Autodesk Inventor part; units mm, degrees
ref_plane "Work Plane1" through (-21.8189, 29, 8.1) normal (0, 1, 0) x (0, 0, 1)
ref_plane "Work Plane2" through (-21.8189, 19, 8.1) normal (0, 0, -1) x (0, 1, 0)
ref_plane "YZ Plane" through (0, 0, 0) normal (1, 0, 0) x (0, 1, 0)
sketch "Sketch1" plane through (0, 0, 0) normal (0, 0, 1) x (1, 0, 0)
  line L0 (5.8439, -14.5) -> (6.8, -14.5)
  line L1 (6.8, -5.5) -> (6.8, -14.5)
  line L2 (6.8, -5.5) -> (5.8439, -5.5)
  arc A0 (5.8439, -3.1) -> (5.8439, -5.5) centre (4, -4.3) ccw
  line L3 (5.8439, -3.1) -> (6.8, -3.1)
  line L4 (6.8, 0) -> (6.8, -3.1)
  line L5 (0, 0) -> (6.8, 0)
  line L6 (0, -20) -> (0, 0)
  line L7 (0, -20) -> (6.8, -20)
  line L8 (6.8, -16.9) -> (6.8, -20)
  line L9 (6.8, -16.9) -> (5.8439, -16.9)
  arc A1 (5.8439, -14.5) -> (5.8439, -16.9) centre (4, -15.7) ccw
  line L10 (-47.1, -14.5) -> (-46.1439, -14.5)
  arc A2 (-46.1439, -16.9) -> (-46.1439, -14.5) centre (-44.3, -15.7) ccw
  line L11 (-46.1439, -16.9) -> (-47.1, -16.9)
  line L12 (-47.1, -16.9) -> (-47.1, -20)
  line L13 (-40.3, -20) -> (-47.1, -20)
  line L14 (-40.3, 0) -> (-40.3, -20)
  line L15 (-40.3, 0) -> (-47.1, 0)
  line L16 (-47.1, 0) -> (-47.1, -3.1)
  line L17 (-47.1, -3.1) -> (-46.1439, -3.1)
  arc A3 (-46.1439, -5.5) -> (-46.1439, -3.1) centre (-44.3, -4.3) ccw
  line L18 (-46.1439, -5.5) -> (-47.1, -5.5)
  line L19 (-47.1, -5.5) -> (-47.1, -14.5)
extrude "Extrusion1" add sketch "Sketch1" along normal blind 4
sketch "Sketch2" plane through (0, 0, 0) normal (0, 1, 0) x (1, 0, 0)
  line L0 (0, 0) -> (6.8, 0)
  line L1 (0, 0) -> (0, -4)
  line L2 (6.8, -4) -> (0, -4)
  line L3 (6.8, 0) -> (6.8, -4)
  line L4 (-47.1, 0) -> (-47.1, -4)
  line L5 (-40.3, -4) -> (-47.1, -4)
  line L6 (6.8, 0) -> (-47.1, 0)
  line L7 (-47.1, 0) -> (-47.1, -4)
  line L8 (-47.1, -4) -> (6.8, -4)
  line L9 (6.8, -4) -> (6.8, 0)
extrude "Extrusion2" add sketch "Sketch2" along normal blind 4 contours L1 L8 L5 L4 L6
sketch "Sketch3" plane through (0, 0, 4) normal (1, 0, 0) x (0, 0, -1)
  line L0 (4, 0) -> (0, 0)
  line L1 (4, 4) -> (4, 0)
  line L2 (0, 4) -> (4, 4)
  line L3 (0, 0) -> (0, 4)
extrude "Extrusion3" add sketch "Sketch3" along normal up to surface (6.8 mm away)
sketch "Sketch4" plane through (0, 4, 0) normal (0, 1, 0) x (1, 0, 0)
  line L0 (6.8, 0) -> (-47.1, 0)
  line L1 (-47.1, -4) -> (6.8, -4)
  line L2 (-9.3767, -8.1) -> (-9.3767, -13.1) construction
  line L3 (-21.8189, -8.1) -> (-9.3767, -8.1) construction
  arc A0 (-17.3767, -8.1) -> (-40.8, 16.4941) centre (-48.3, -14.1) ccw construction
  line L4 (-9.3767, -4) -> (-16.3767, -4) construction
  line L5 (-16.3767, -4) -> (-16.3767, -8.1) construction
  line L6 (-16.3767, -8.1) -> (-9.3767, -8.1) construction
  line L7 (-9.3767, -8.1) -> (-9.3767, -4) construction
  line L8 (-9.3767, -4) -> (-16.3767, -4)
  line L9 (-16.3767, -4) -> (-16.3767, 0)
  line L10 (-16.3767, 0) -> (-9.3767, 0)
  line L11 (-9.3767, 0) -> (-9.3767, -4)
  point P0 (0, 0)
  dimension "d6" = 7
ref_plane "Work Plane1" through (-21.8189, 29, 8.1) normal (0, 1, 0) x (0, 0, 1)
extrude "Extrusion4" add sketch "Sketch4" along normal up to surface (25 mm away)
sketch "Sketch5" plane through (0, 0, 4) normal (0, 0, 1) x (1, 0, 0)
  circle A0 centre (-13.3767, 24) radius 2 construction
  line L0 (-21.8189, 24) -> (-17.3767, 24) construction
  line L1 (-21.8189, 24) -> (-21.8189, 29) construction
  line L2 (-21.8189, 29) -> (-9.3767, 29) construction
  line L3 (-9.3767, 19) -> (-9.3767, 29) construction
  line L4 (-17.3767, 19) -> (-9.3767, 19) construction
  line L5 (-17.3767, 24) -> (-17.3767, 19) construction
  line L6 (-9.3767, 19) -> (-16.3767, 19) construction
  line L7 (-16.3767, 19) -> (-16.3767, 29) construction
  line L8 (-16.3767, 29) -> (-9.3767, 29) construction
  line L9 (-9.3767, 29) -> (-9.3767, 19) construction
  line L10 (-9.3767, 19) -> (-16.3767, 19)
  line L11 (-16.3767, 19) -> (-16.3767, 29)
  line L12 (-16.3767, 29) -> (-9.3767, 29)
  line L13 (-9.3767, 29) -> (-9.3767, 19)
  circle A1 centre (-13.3767, 24) radius 2
ref_plane "Work Plane2" through (-21.8189, 19, 8.1) normal (0, 0, -1) x (0, 1, 0)
extrude "Extrusion5" add sketch "Sketch5" along normal up to surface (4.1 mm away)
sketch "Sketch6" plane through (-16.3767, 19, 8.1) normal (-1, 0, 0) x (0, 0, 1)
  line L0 (0, 5) -> (-24.5941, 5) construction
  line L1 (0, 0) -> (-24.5941, 0) construction
  line L2 (-8.1, 10) -> (0.5132, 10) construction
  line L3 (0.5132, 10) -> (0.5132, 5) construction
  line L4 (0.5132, 5) -> (-8.1, 5) construction
  line L5 (-8.1, 5) -> (-8.1, 10) construction
  line L6 (-8.1, 10) -> (0, 10)
  line L7 (0, 10) -> (0, 5)
  line L8 (0, 5) -> (-8.1, 5)
  line L9 (-8.1, 5) -> (-8.1, 10)
  point P0 (-8.1, -19)
extrude "Extrusion6" add sketch "Sketch6" along normal blind 5
sketch "Sketch7" plane through (-16.3767, 24, 0) normal (0, -1, 0) x (1, 0, 0)
  line L0 (0, 8.1) -> (0, 0)
  line L1 (0, 8.1) -> (-5, 8.1)
  line L2 (-5, 0) -> (-5, 8.1)
  line L3 (0, 0) -> (-5, 0)
  point P0 (16.3767, 0)
extrude "Extrusion7" cut sketch "Sketch7" against normal blind 0.4
sketch "Sketch8" plane through (0, 0, 0) normal (0, 0, -1) x (-1, 0, 0)
  circle A0 centre (13.3767, 24) radius 2 construction
  circle A1 centre (13.3767, 24) radius 2
extrude "Extrusion8" cut sketch "Sketch8" against normal blind 4
fillet "Fillet3" radius 1 1 edges at (-16.3767, 24.4, 4.05)
sketch "Sketch9" plane through (-9.3767, 19, 8.1) normal (1, 0, 0) x (0, 0, -1)
  line L0 (0, 0) -> (0, 10)
  line L1 (8.1, 7) -> (0, 7) construction
  line L2 (8.1, 3) -> (0, 3) construction
  line L3 (24.5941, 5) -> (0, 5) construction
  line L4 (-5, 5) -> (0, 5) construction
  line L5 (4, 8.75) -> (7.5, 8.75)
  line L6 (7.5, 8.75) -> (7.5, 1.25)
  line L7 (7.5, 1.25) -> (4, 1.25)
  line L8 (4, 1.25) -> (4, 8.75)
  point P0 (8.1, -19)
  point P1 (4, 5)
  dimension "d20" = 3.5
  dimension "d21" = 7.5
  dimension "d22" = 4
extrude "Extrusion9" cut sketch "Sketch9" against normal blind 7.5
sketch "Sketch10" plane through (-16.3767, 19, 4) normal (0, -1, 0) x (1, 0, 0)
  line L0 (0, 4.1) -> (7, 4.1)
  line L1 (0, 0) -> (0, 4.1)
  line L2 (7, 0) -> (0, 0)
  line L3 (7, 0) -> (7, 4.1)
  point P0 (16.3767, -4)
extrude "Extrusion10" add sketch "Sketch10" along normal blind 3
fillet "Fillet4" radius 3 1 edges at (-12.8767, 16, 4)
sketch "Sketch11" plane through (0, 0, 0) normal (0, -1, 0) x (1, 0, 0)
  line L0 (-40.3, 0) -> (-40.3, 4)
  line L1 (0, 0) -> (-40.3, 0)
  line L2 (0, 0) -> (0, 4)
  line L3 (-40.3, 4) -> (0, 4)
extrude "Extrusion11" cut sketch "Sketch11" against normal blind 0.3
sketch "Sketch12" plane through (0, -20, 0) normal (-1, 0, 0) x (0, 0, 1)
  line L0 (0, 0) -> (0, 20.3)
  line L1 (0, 0) -> (4, 0)
  line L2 (4, 20.3) -> (4, 0)
  line L3 (4, 20.3) -> (0, 20.3)
  point P0 (0, 20)
extrude "Extrusion12" cut sketch "Sketch12" against normal blind 0.3
sketch "Sketch13" plane through (-40.3, -20, 4) normal (1, 0, 0) x (0, 0, -1)
  line L0 (4, 0) -> (4, 20.3)
  line L1 (4, 20.3) -> (0, 20.3)
  line L2 (0, 0) -> (0, 20.3)
  line L3 (4, 0) -> (0, 0)
  point P0 (4, 20)
extrude "Extrusion13" cut sketch "Sketch13" against normal blind 0.3
fillet "Fillet5" radius 1 2 edges at (6.8, 4, 2) (-47.1, 4, 2)
sketch "Sketch15" plane through (0, 0, 0) normal (0, 0, -1) x (-1, 0, 0)
  circle A0 centre (13.3767, 24) radius 2
  line L0 (9.3767, 29) -> (21.3767, 29)
  line L1 (21.3767, 29) -> (21.3767, 7.8113)
  line L2 (21.3767, 7.8113) -> (9.3767, 7.8113)
  line L3 (9.3767, 7.8113) -> (9.3767, 29)
  point P0 (0, 0)
extrude "Extrusion14" cut sketch "Sketch15" against normal through all
properties part number "MG996RBracketTop"
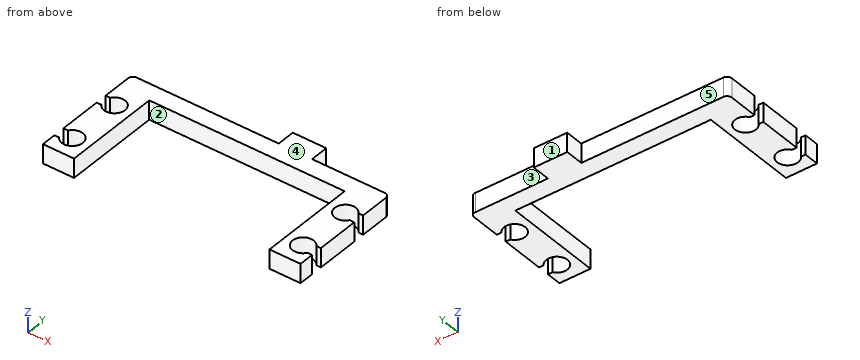
Could you check a few things on this model? Use its own coordinates, in mm. Face numbers are marked on the shaded views. A direction names the side the tool comes from. Round coordinates to 2 decimals unless told otherwise and drop trailing zeros. Order: outer loops, then holes, each group sorted by start corner. A loop starts at its lowest first (then second) coordinate and runs counter-clockwise, first axis right, second up. Notation, with made-up numbers: M -36.75,-26 L -32.75,-26 A14 ccw -32.75,-13 Z; hole C -34.5,-31 d2. An arc over 180 degrees is marked long. One line per item, written item: value.
(1) Imagine slicing it at B-B (x = -44.3). Write out the boundary of the cut face in (y, z), and give its area (3 significant figures).
Ans:
outline: M -20,0 L -17.9,0 L -17.9,4 L -20,4 Z; M -13.5,0 L -6.5,0 L -6.5,4 L -13.5,4 Z; M -2.1,0 L 4,0 L 4,4 L -2.1,4 Z
area: 60.8 mm^2
(2) Imagine slicing it at A-A (y = -4.3). Write out the boundary of the cut face in (x, z), and give its area (3 significant figures).
Ans:
outline: M -42.1,0 L -40.6,0 L -40.6,4 L -42.1,4 Z; M 0.3,0 L 1.8,0 L 1.8,4 L 0.3,4 Z
area: 12.0 mm^2
(3) Which directions (+Z, -Z, +X, -X, +Y, -Y) give clear straight access to the entire face, cutting with the end or side of a thin tool? Please do the marked faces 3, 4 and 5.
Ans:
face 3: +Z, -Z, +X, +Y
face 4: +Z, +X, -X, +Y, -Y
face 5: +Z, -Z, -X, +Y
(4) I need wall thicknesses on line 1 along Y through (x, z) = (-44.3, 2.65); line 2 along X through (y, z) = (-4.3, 2); line 3 along X through (y, z) = (-11.5, 0.95). Which ranges of each line are inside material? Lowest first, please. Write a range as from..to.
Ans:
line 1: y = -20..-17.9, -13.5..-6.5, -2.1..4
line 2: x = -42.1..-40.6, 0.3..1.8
line 3: x = -47.1..-40.6, 0.3..6.8
(5) If we mould it in two halves opening along X, with no side actions, what happens to the marked faces 1 and 2? For each: released by +X, released by -X, zero draft, split by the parting line, or undercut.
Ans:
face 1: zero draft
face 2: undercut
(6) Imagine slicing it at D-D (y = -8.5). Write out the boundary of the cut face in (x, z).
Ans:
outline: M -47.1,0 L -40.6,0 L -40.6,4 L -47.1,4 Z; M 0.3,0 L 6.8,0 L 6.8,4 L 0.3,4 Z
(7) I'm going to push flat-ended pins straight in: P1, Ø5, axis at x = 4, y = -15.7, coming from the -Z side; P2, Ø0.8, axis at x = 6.5, z = 1.5, coming from the +Y side; P3, Ø1.5, axis at x = -21.5, y = -1.5, coming from the +Z side; P4, Ø1.1, axis at y = 6, z = 2, coming from the -X side. Where does each tip first touch, or does it pass through?
Ans:
P1: stops at z = 0
P2: stops at y = 3.95
P3: passes through
P4: stops at x = -16.38
